```python
from build123d import *

# Parameters (mm, degrees)
SKETCH2_W           = 78.150454931
SKETCH2_H           = 77.221988429
SKETCH2_R           = 2.413
SKETCH2_W_2         = 35.652738644
SKETCH2_H_2         = 57.874285637
BOSS_EXTRUDE1_DEPTH = 2.54
SKETCH3_W           = 2.159598277
SKETCH3_H           = 77.221988429
BOSS_EXTRUDE2_DEPTH = 17.78
SKETCH5_R           = 2.54
CUT_EXTRUDE2_DEPTH  = 17.78


with BuildPart() as part:
    # Sketch2 → Boss-Extrude1 (new body)
    with BuildSketch(Plane.XY):
        with Locations((6.487490533, -7.63692736)):
            Rectangle(SKETCH2_W, SKETCH2_H)
        with Locations((-26.23773696, 22.67645588)):
            Circle(SKETCH2_R, mode=Mode.SUBTRACT)
        with Locations((37.26226304, 22.67645588)):
            Circle(SKETCH2_R, mode=Mode.SUBTRACT)
        with Locations((37.26226304, -37.64854412)):
            Circle(SKETCH2_R, mode=Mode.SUBTRACT)
        with Locations((-26.23773696, -37.64854412)):
            Circle(SKETCH2_R, mode=Mode.SUBTRACT)
        with Locations((4.092128919, -8.801242849)):
            Rectangle(SKETCH2_W_2, SKETCH2_H_2, mode=Mode.SUBTRACT)
    extrude(amount=BOSS_EXTRUDE1_DEPTH)

    # Sketch3 → Boss-Extrude2 (add)
    with BuildSketch(Plane.XY.offset(2.54)):
        with Locations((-31.507937795, -7.63692736)):
            Rectangle(SKETCH3_W, SKETCH3_H)
    extrude(amount=BOSS_EXTRUDE2_DEPTH)

    # Sketch5 → Cut-Extrude2 (cut)
    with BuildSketch(Plane(origin=(-30.428138656, 0, 0), x_dir=(0, 0, -1), z_dir=(1, 0, 0))):
        with Locations((-11.43, -7.636927359)):
            Circle(SKETCH5_R)
        with Locations((-11.43, 11.668569748)):
            Circle(SKETCH5_R)
        with Locations((-11.43, -26.942424466)):
            Circle(SKETCH5_R)
    extrude(amount=-CUT_EXTRUDE2_DEPTH, mode=Mode.SUBTRACT)


solid = part.part
```
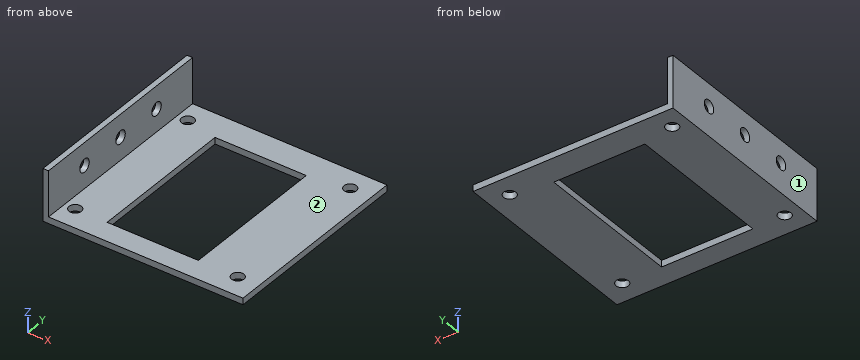
Geometry check sheet. Reference: the model listing, model coordinates, mm. Face numbers are marked on the shaded views. A direction names the side the tool comes from. Coordinates: 2 decimals unless noted, no trailing zeros. Write each loop counter-clockwise with the first axis right and the second up, starting at its lowest first coordinate (ties: lowest second). Pieces come first, ordered by that corner, then holes. Notation, with made-up numbers: M -4,35.5 L 24,35.5 A17 cw 24,46.5 Z; hole C 64,-19.75 d7. An arc over 180 degrees is marked long. One line per item, written item: value. Start each with the question number.
(1) Sectioned sample at B-B, the plane y = -17. Enter the section's corners in (x, z), and give its area (3 significant figures).
(2) Sectioned sample at A-A, the plane z = 11.43. Enter the section's corners in (x, y).
(3) Sectioned sample at C-C, the plane x = -25.5. Enter the section's corners in (y, z).
(4) Scan lines: line 1 along Y through (x, z) = (-30.95, 11.43); line 2 along Y through (x, z) = (6, 2.5); line 3 along X through (y, z) = (-24, 2.5). Record each from-to range of solid material in increasing order. Write a range as [from, to].
(5) Sectioned sample at D-D, the plane x = -5. Enter the section's corners in (y, z), and give its area (3 significant figures).
(6) Tool access check on the marked faces 1 and 2. Record the directions out of +Z, -Z, +X, -X, +Y, -Y that give a thin tool (end or side, any length) a straight path to the whole face; none if there is none.
(7) Depth check by flat-ended pin: pin 1 (6 mm diameter, centred on y = 13, z = 17, fed in from +X); pin 2 (6.5 mm diameter, centred on x = 37.26, y = 22.68, fed in from -Z); pin 3 (6.5 mm diameter, centred on x = -26.24, y = 22.68, fed in from +Z). Enter the tip coordinate at first touch or a pass-through.
Filled sheet:
1. outline: M -32.59,0 L -13.73,0 L -13.73,2.54 L -30.43,2.54 L -30.43,20.32 L -32.59,20.32 Z; M 21.92,0 L 45.56,0 L 45.56,2.54 L 21.92,2.54 Z
1. area: 146 mm²
2. outline: M -32.59,-46.25 L -30.43,-46.25 L -30.43,-29.48 L -32.59,-29.48 Z; M -32.59,-24.4 L -30.43,-24.4 L -30.43,-10.18 L -32.59,-10.18 Z; M -32.59,-5.1 L -30.43,-5.1 L -30.43,9.13 L -32.59,9.13 Z; M -32.59,14.21 L -30.43,14.21 L -30.43,30.97 L -32.59,30.97 Z
3. outline: M -46.25,0 L -39.95,0 L -39.95,2.54 L -46.25,2.54 Z; M -35.35,0 L 20.38,0 L 20.38,2.54 L -35.35,2.54 Z; M 24.97,0 L 30.97,0 L 30.97,2.54 L 24.97,2.54 Z
4. line 1: [-46.25, -29.48], [-24.4, -10.18], [-5.1, 9.13], [14.21, 30.97]
4. line 2: [-46.25, -37.74], [20.14, 30.97]
4. line 3: [-32.59, -13.73], [21.92, 45.56]
5. outline: M -46.25,0 L -37.74,0 L -37.74,2.54 L -46.25,2.54 Z; M 20.14,0 L 30.97,0 L 30.97,2.54 L 20.14,2.54 Z
5. area: 49.1 mm²
6. face 1: +Z, -Z, -X, +Y, -Y
6. face 2: +Z, +X, +Y, -Y
7. pin 1: x = -30.43
7. pin 2: z = 0
7. pin 3: z = 2.54
